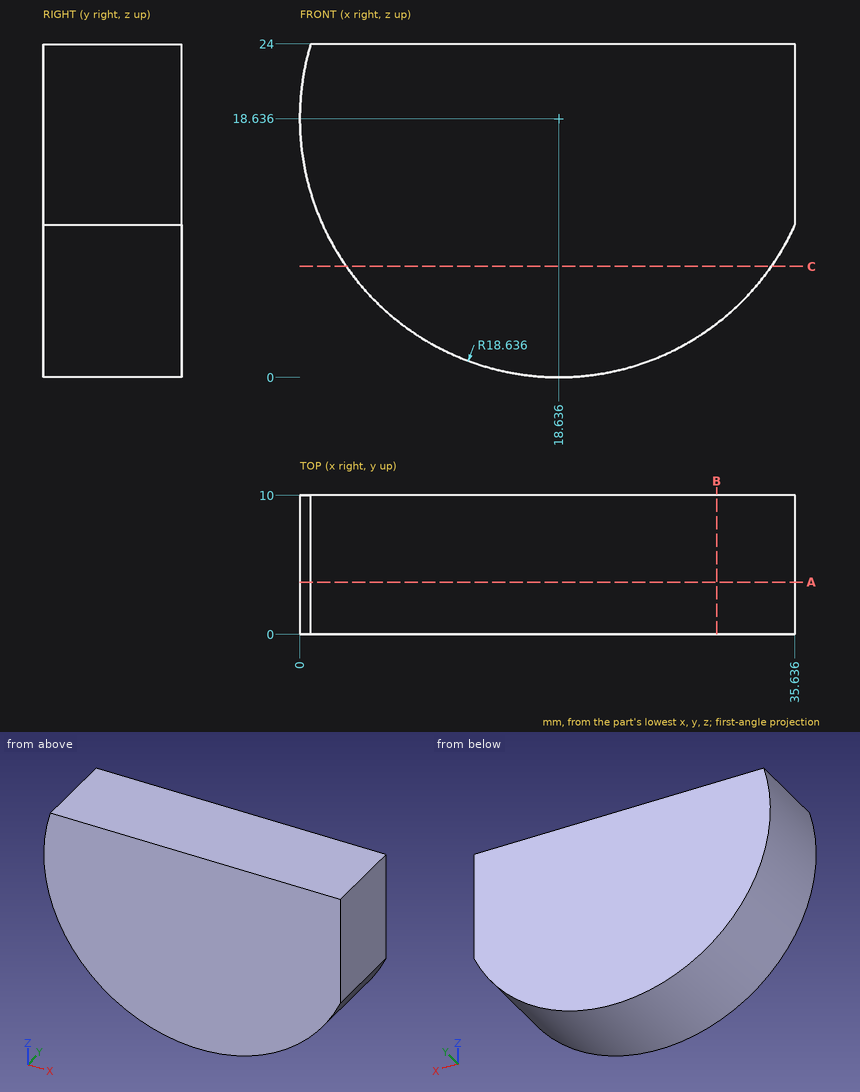
The drawing under review shows one solid part. Ordinate dimensions are in mm from its lowest x, y, z. Round coordinates to 2 decimals unless told otherwise and drop trailing zeros. Write each loop counter-clockwise with the first axis right and the second up, starting at its lowest first coordinate (ties: lowest second). Pieces come first, ordered by that corner, then holes. Notation, with made-up numbers: (2.25, 23.5) - (31.25, 23.5) arc R21 cw to (31.25, 59.5) - close; hole circle Ø11 at (8.5, 25). An arc over 180 degrees is marked (long way). Use one line per item in the form item = value.
Q1. Consider section B-B (x = 30). State the section outline as (y, z) points (1 decimal), and give its area (3 significant figures).
Answer key:
outline = (0, 3.9) - (10, 3.9) - (10, 24) - (0, 24) - close
area = 201 mm2
Q2. Consider section C-C (z = 8). State the section outline as (x, y) points, and give its area (3 significant figures).
Answer key:
outline = (3.33, 0) - (33.94, 0) - (33.94, 10) - (3.33, 10) - close
area = 306 mm2
Q3. For line 1 (X direction, y = 9.5, z = 18.25); line 2 (X direction, y = 4.25, z = 7.75); line 3 (Z direction, x = 19, y = 4.5), list the stretches that pass through material, from the lowest coordinate up. Write a range as [from, to].
Answer key:
line_1 = [0, 35.64]
line_2 = [3.51, 33.76]
line_3 = [0, 24]
Q4. Consider section A-A (y = 3.75). State the section outline as (x, z) points, and give its area (3 significant figures).
Answer key:
outline = (0.79, 24) arc R18.64 ccw to (35.64, 11) - (35.64, 24) - close
area = 727 mm2
